Read the model definition and answer for the solid it produces. Units are mm, in the model's axes. A direction names the side the tool comes from. Coordinates: 2 decimals unless noted, no trailing zeros. Write each loop counter-clockwise with the first axis right and the second up, starting at its lowest first coordinate (ties: lowest second). Pieces come first, ordered by that corner, then holes.
1) The part is cut by section B-B (y = -42). Determine the outline of the cut face in (x, z).
2) The part is cut by section A-A (x = 176.5). Determine the outline of the cut face in (y, z).
3) Find the intervals of material crossed by line 1 (Z direction, x = 7.5, y = -18.5); line 2 (X direction, y = -30.5, z = 28); line 3 (Z direction, x = 37, y = -10), in increasing order.
4) Which of the six approach directions +Z, -Z, +X, -X, +Y, -Y give full straight-line access (tool end or side, diameter ignored) to faces 5 (the face through (197, -25, 58)), 6 (the face through (3, -25, 30))?
5) Determine the mould class of faces 1 (the face through (3, -25, 58)), 2 (the face through (10.5, -25, 7)), 3 (the face through (99, -25, 60)), 4 (the face through (10.5, -25, 53)) for opening direction X: +X half, -X half, draft (parallel to the pull), parting line (faces both ways), or undercut.
6) The part is cut by section C-C (z = 29). Determine the outline of the cut face in (x, y), then the cut area to 3 significant figures.
from build123d import *

# Parameters (mm, degrees)
SKETCH_W     = 200
SKETCH_H     = 60
PAD_DEPTH    = 50
CHAMFER_SIZE = 5
SKETCH001_R  = 1.5
POCKET_DEPTH = 50.001


with BuildPart() as part:
    # Sketch → Pad (new body)
    with BuildSketch(Plane.XZ):
        with Locations((100, 30)):
            Rectangle(SKETCH_W, SKETCH_H)
    extrude(amount=PAD_DEPTH)

    # Chamfer
    chamfer_edges = [part.edges().sort_by_distance(p)[0] for p in [
        (200, -25, 0),
        (200, -25, 60),
        (0, -25, 60),
        (0, -25, 0),
    ]]
    chamfer(chamfer_edges, length=CHAMFER_SIZE)

    # Sketch001 (on Face5 of Chamfer) → Pocket (cut, through all)
    with BuildSketch(Plane.XZ.offset(50)):
        with Locations((7.5, 52.5)):
            Circle(SKETCH001_R)
        with Locations((192.5, 52.5)):
            Circle(SKETCH001_R)
        with Locations((192.5, 7.5)):
            Circle(SKETCH001_R)
        with Locations((7.5, 7.5)):
            Circle(SKETCH001_R)
        Polygon((10.5, 57), (189.5, 57), (189.5, 49.5), (197, 49.5), (197, 10.5), (189.5, 10.5), (189.5, 3), (10.5, 3), (10.5, 10.5), (3, 10.5), (3, 49.5), (10.5, 49.5), align=None)
    extrude(amount=-POCKET_DEPTH, mode=Mode.SUBTRACT)


solid = part.part
Reported:
1. outline: (0, 5) - (5, 0) - (195, 0) - (200, 5) - (200, 55) - (195, 60) - (5, 60) - (0, 55) - close; hole (3, 10.5) - (10.5, 10.5) - (10.5, 3) - (189.5, 3) - (189.5, 10.5) - (197, 10.5) - (197, 49.5) - (189.5, 49.5) - (189.5, 57) - (10.5, 57) - (10.5, 49.5) - (3, 49.5) - close; hole circle Ø3 at (7.5, 7.5); hole circle Ø3 at (7.5, 52.5); hole circle Ø3 at (192.5, 7.5); hole circle Ø3 at (192.5, 52.5)
2. outline: (-50, 0) - (0, 0) - (0, 3) - (-50, 3) - close; (-50, 57) - (0, 57) - (0, 60) - (-50, 60) - close
3. line 1: z = 0 to 6, 9 to 10.5, 49.5 to 51, 54 to 60
3. line 2: x = 0 to 3, 197 to 200
3. line 3: z = 0 to 3, 57 to 60
4. face 5: +Z, +X, +Y, -Y
4. face 6: +Y, -Y
5. face 1: -X half
5. face 2: undercut
5. face 3: draft
5. face 4: undercut
6. outline: (0, -50) - (3, -50) - (3, 0) - (0, 0) - close; (197, -50) - (200, -50) - (200, 0) - (197, 0) - close
6. area: 300 mm2
